Check sheet for the modelled part. Datum: model origin and axes. Units: mm. Face numbers are marked on the shaded views. A direction names the side the tool comes from. Give positions to 0.01 mm unless a question says otherwise; leave off trailing zeros. Order: outer loops, then holes, each group sorted by start corner. A loop starts at its lowest first (then second) coordinate and runs counter-clockwise, first axis right, second up. Notation, with made-up numbers: M -33.75,27 L -3.75,27 A23 ccw -3.75,43 Z; hole C -16.75,13 d3. An arc over 180 degrees is marked long. Return JSON: item names as keys, results as strings. Group by question number.
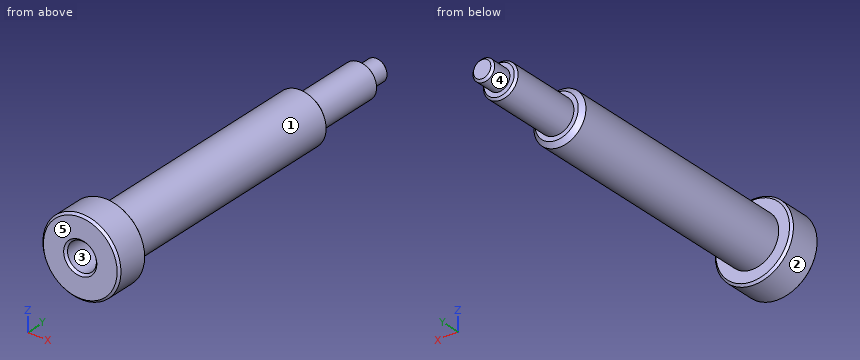
Solid Edge part; units mm, degrees
sketch "Sketch1" plane through (0, 0, 0) normal (0, -1, 0) x (1, 0, 0)
  circle A0 centre (0, 0) radius 6
extrude "Protrusion1" add sketch "Sketch1" along normal mid plane 80
sketch "Sketch2" plane through (0, -40, 0) normal (0, -1, 0) x (1, 0, 0)
  circle A0 centre (0, 0) radius 9
extrude "Ausprägung_2" add sketch "Sketch2" along normal blind 8
sketch "Sketch3" plane through (0, 40, 0) normal (0, 1, 0) x (1, 0, 0)
  circle A0 centre (0, 0) radius 2.5
extrude "Ausschnitt_1" cut sketch "Sketch3" against normal blind 5 flip side to cut
sketch "Sketch4" plane through (0, 35, 0) normal (0, 1, 0) x (0, 0, -1)
  circle A0 centre (0, 0) radius 4
extrude "Ausschnitt_2" cut sketch "Sketch4" against normal blind 17 flip side to cut
cosmetic_thread "Gewinde_1" thread depth 4
chamfer "Fase_1" distance 0.5 angle 45 1 edges at (-2.5, 40, 0)
chamfer "Fase_2" distance 1 angle 45 1 edges at (0, 18, -6)
cosmetic_thread "Gewinde_2" thread depth 15
chamfer "Fase_3" distance 0.5 angle 45 1 edges at (0, 35, 4)
hole "Bohrung_1" at (0, -48, 0) direction (0, 1, 0) diameter 6.647 depth 24 thread major 8 thread length 2
chamfer "Fase_4" distance 0.5 angle 45 1 edges at (0, -48, 3.3235)
chamfer "Fase_5" distance 0.5 angle 45 2 edges at (-9, -48, 0) (-9, -40, 0)
1) Release check for a two-part mould opening along Z. For the marked faces 3, 4 and 5 record: released by +Z, released by -Z, zero draft, split by the parting line, or undercut.
2) Sectioned sample at C-C on y = -29. Record the boundary of the cut face in (x, z), then the cut area to 3 significant figures.
3) Sectioned sample at D-D on y = 30. Record the boundary of the cut face in (x, z), then the cut area to 3 significant figures.
4) Material ranges on line 1 along X through (y, z) = (-31.75, 0); line 2 along Z through (x, y) = (0, -42.25), recorded low to high.
5) Depth check by flat-ended pin: P1, Ø4, axis at x = 0, z = 0, coming from the -Y side; P2, Ø3, axis at x = 7, z = -2, coming from the +Y side; P3, Ø2, axis at x = 6, y = -10, coming from the +Z side. Enter the tip coordinate at first touch or a pass-through.
6) Tool access check on the marked faces 1 and 2. Record the directions out of +Z, -Z, +X, -X, +Y, -Y that give a thin tool (end or side, any length) a straight path to the whole face; none if there is none.
Reply:
{
 "1": {"face 3": "undercut", "face 4": "split by the parting line", "face 5": "zero draft"},
 "2": {"outline": "C 0,0 d12; hole C 0,0 d6.65", "area": "78.4 mm^2"},
 "3": {"outline": "C 0,0 d8", "area": "50.3 mm^2"},
 "4": {"line 1": "-6 to -3.32, 3.32 to 6", "line 2": "-9 to -3.32, 3.32 to 9"},
 "5": {"P1": "y = -24", "P2": "y = 17.22", "P3": "z = 3.32"},
 "6": {"face 1": "+Y", "face 2": "+Y, -Y"}
}
